Build history of the part. All positions in model axes, mm. Face numbers are marked on the shaded views. A direction names the side the tool comes from. Round coordinates to 2 decimals unless told otherwise and drop trailing zeros. Write each loop counter-clockwise with the first axis right and the second up, starting at its lowest first coordinate (ties: lowest second). Pieces come first, ordered by that corner, then holes. Notation, with made-up numbers: (-25.75, 14.5) -> (-3.75, 14.5) arc R23 ccw to (-3.75, 27.5) -> close; hole circle Ø8 at (-27.5, 23.25). An arc over 180 degrees is marked (long way). Answer as CSV lines item,"result".
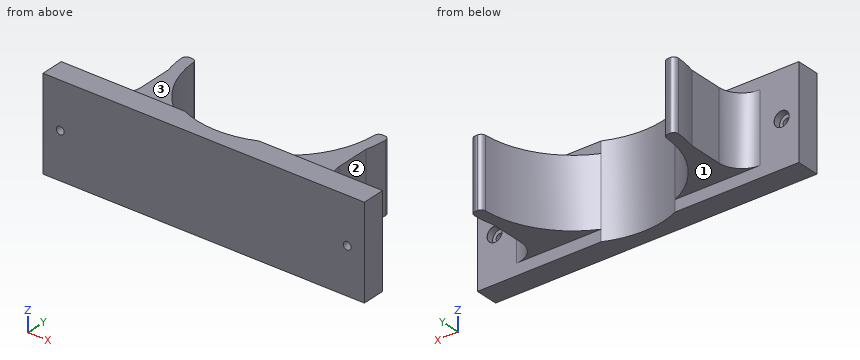
from build123d import *

# Parameters (mm, degrees)
BOSS_EXTRUDE3_DEPTH           = 20
BOSS_EXTRUDE3_DEPTH_BACK      = 20
BOSS_EXTRUDE4_DEPTH           = 15
BOSS_EXTRUDE4_DEPTH_BACK      = 15
BOSS_EXTRUDE5_DEPTH           = 15
BOSS_EXTRUDE5_DEPTH_BACK      = 15
FILLET1_R                     = 10
CBORE_FOR_M3_SHCS1_AT_2_COUNT = 2
CBORE_FOR_M3_SHCS1_AT_2_PITCH = 125
FILLET2_R                     = 2


with BuildPart() as part:
    # Sketch1 → Boss-Extrude3 (new, two sides: drawn at the far end of the back side and taken through both)
    with BuildSketch(Plane.XY.offset(-BOSS_EXTRUDE3_DEPTH_BACK)):
        with BuildLine():
            Line((-43.065388601, -36.056178761), (-70, -36.056178761))
            Line((-70, -36.056178761), (-70, -46.056178761))
            Line((-70, -46.056178761), (70, -46.056178761))
            Line((70, -46.056178761), (70, -36.056178761))
            Line((70, -36.056178761), (43.065388601, -36.056178761))
            Line((43.065388601, -36.056178761), (26.080681992, -36.056178761))
            Line((26.080681992, -36.056178761), (16.130777202, -36.056178761))
            ThreePointArc((16.130777202, -36.056178761), (0, -39.5), (-16.130777202, -36.056178761))
            Line((-16.130777202, -36.056178761), (-26.080681992, -36.056178761))
            Line((-26.080681992, -36.056178761), (-43.065388601, -36.056178761))
        make_face()
    extrude(amount=BOSS_EXTRUDE3_DEPTH + BOSS_EXTRUDE3_DEPTH_BACK)

    # Sketch1_6 → Boss-Extrude4 (add, two sides: drawn at the far end of the back side and taken through both)
    with BuildSketch(Plane.XY.offset(-BOSS_EXTRUDE4_DEPTH_BACK)):
        with BuildLine():
            ThreePointArc((-43.065388601, -11.208135645), (-36.737597653, -25.111728708), (-26.080681992, -36.056178761))
            Line((-26.080681992, -36.056178761), (-16.130777202, -36.056178761))
            ThreePointArc((-16.130777202, -36.056178761), (-33.146762281, -21.483532071), (-39.5, 0))
            Line((-39.5, 0), (-44.5, 0))
            ThreePointArc((-44.5, 0), (-44.139890081, -5.649787927), (-43.065388601, -11.208135645))
        make_face()
        with BuildLine():
            ThreePointArc((39.5, 0), (33.146762281, -21.483532071), (16.130777202, -36.056178761))
            Line((16.130777202, -36.056178761), (26.080681992, -36.056178761))
            ThreePointArc((26.080681992, -36.056178761), (36.737597653, -25.111728708), (43.065388601, -11.208135645))
            ThreePointArc((43.065388601, -11.208135645), (44.139890081, -5.649787927), (44.5, 0))
            Line((44.5, 0), (39.5, 0))
        make_face()
    extrude(amount=BOSS_EXTRUDE4_DEPTH + BOSS_EXTRUDE4_DEPTH_BACK)

    # Sketch1_7 → Boss-Extrude5 (add, two sides: drawn at the far end of the back side and taken through both)
    with BuildSketch(Plane.XY.offset(-BOSS_EXTRUDE5_DEPTH_BACK)):
        with BuildLine():
            Line((26.080681992, -36.056178761), (43.065388601, -36.056178761))
            Line((43.065388601, -36.056178761), (43.065388601, -11.208135645))
            ThreePointArc((43.065388601, -11.208135645), (36.737597653, -25.111728708), (26.080681992, -36.056178761))
        make_face()
        with BuildLine():
            Line((-43.065388601, -11.208135645), (-43.065388601, -36.056178761))
            Line((-43.065388601, -36.056178761), (-26.080681992, -36.056178761))
            ThreePointArc((-26.080681992, -36.056178761), (-36.737597653, -25.111728708), (-43.065388601, -11.208135645))
        make_face()
    extrude(amount=BOSS_EXTRUDE5_DEPTH + BOSS_EXTRUDE5_DEPTH_BACK)

    # Fillet1
    fillet1_edges = [part.edges().sort_by_distance(p)[0] for p in [
        (43.065388601, -36.056178761, 0),
        (-43.065388601, -36.056178761, 0),
    ]]
    fillet(fillet1_edges, radius=FILLET1_R)

    # Sketch4 → CBORE for M3 SHCS1 (revolve, cut)
    with BuildSketch(Plane(origin=(-62.5, -36.056178761, 0), x_dir=(0, 0, 1), z_dir=(1, 0, 0))):
        Polygon((0, 0), (0, 10), (1.7, 10), (1.7, 3), (3.25, 3), (3.25, 0.025), (3.275, 0), align=None)
    cbore_for_m3_shcs1 = revolve(axis=Axis((-62.5, -29.706178761, 0), (0, -1, 0)), mode=Mode.SUBTRACT)

    # CBORE for M3 SHCS1 at 2: CBORE for M3 SHCS1 ×2
    with Locations(*[(i * CBORE_FOR_M3_SHCS1_AT_2_PITCH, 0, 0) for i in range(1, CBORE_FOR_M3_SHCS1_AT_2_COUNT)]):
        add(cbore_for_m3_shcs1, mode=Mode.SUBTRACT)

    # Fillet2
    fillet2_edges = [part.edges().sort_by_distance(p)[0] for p in [
        (-44.5, 0, 0),
        (-39.5, 0, 0),
        (44.5, 0, 0),
        (39.5, 0, 0),
    ]]
    fillet(fillet2_edges, radius=FILLET2_R)


solid = part.part
1. Which spindle directions (+Z, -Z, +X, -X, +Y, -Y) get a long thin tool onto all of the face, cutting with end or side? Do the marked faces 1, 2 and 3. Say none if no direction does.
Results found:
face 1,"-Z, +X, -X, +Y"
face 2,"+Z, -Z, +X"
face 3,"+Z, +X, -X, +Y"
2. Cut at A-A, the plane x = 62.5. Write the cut outline in (y, z) (3 decimals), then the cut area to 3 significant figures.
Results found:
outline,"(-46.056, -20) -> (-36.056, -20) -> (-36.056, -3.275) -> (-36.081, -3.25) -> (-39.056, -3.25) -> (-39.056, -1.7) -> (-46.056, -1.7) -> close; (-46.056, 1.7) -> (-39.056, 1.7) -> (-39.056, 3.25) -> (-36.081, 3.25) -> (-36.056, 3.275) -> (-36.056, 20) -> (-46.056, 20) -> close"
area,"357 mm2"
3. Cut at B-B, the plane y = -8. Write the cut outline in (x, z) (3 decimals).
Results found:
outline,"(-43.775, -15) -> (-38.681, -15) -> (-38.681, 15) -> (-43.775, 15) -> close; (38.681, -15) -> (43.775, -15) -> (43.775, 15) -> (38.681, 15) -> close"
4. Cut at C-C, the plane z = 7.5. Write the cut outline in (x, y), then the cut area to 3 significant figures.
Results found:
outline,"(-70, -46.06) -> (70, -46.06) -> (70, -36.06) -> (53.07, -36.06) arc R10 cw to (43.07, -26.06) -> (43.07, -11.21) arc R44.5 ccw to (44.45, -2.09) arc R2 ccw to (42.45, 0) -> (41.45, 0) arc R2 ccw to (39.45, -1.9) arc R39.5 cw to (-39.45, -1.9) arc R2 ccw to (-41.45, 0) -> (-42.45, 0) arc R2 ccw to (-44.45, -2.09) arc R44.5 ccw to (-43.07, -11.21) -> (-43.07, -26.06) arc R10 cw to (-53.07, -36.06) -> (-70, -36.06) -> close"
area,"2,120 mm2"
5. Cut at D-D, the plane z = 0. Count the separate pieces of the cut face and the enclosed holes in it, then the cut area to 3 significant figures.
Results found:
separate pieces,"3"
enclosed holes,"0"
area,"2,030 mm2"
6. Probe line 1 along X through (y, z) = (-40.75, 0); line 2 along Z through (x, y) = (62.5, -41.5); line 3 along Z through (x, y) = (-62.5, -37). List the from-to ranges inside material, lowest first.
Results found:
line 1,"x = -70 to -64.2, -60.8 to 60.8, 64.2 to 70"
line 2,"z = -20 to -1.7, 1.7 to 20"
line 3,"z = -20 to -3.25, 3.25 to 20"
7. Drop flat-ended pins along their axis: pin 1 Ø4 at (y, z) = (-13, -12) entering from +X; pin 2 Ø3 at (x, z) = (-61.5, 0.5) entering from +Y; pin 3 Ø10.5 at (x, z) = (-62.5, 0) entering from +Y. Give the stop position or say it passes through.
Results found:
pin 1,"stops at x = 43.12"
pin 2,"stops at y = -39.06"
pin 3,"stops at y = -36.06"
